Source: CAD feature listing. Evaluate the final solid. Frame: model axes, mm. A direction names the side the tool comes from. Give positions to 0.01 mm unless a question says otherwise; leave off trailing zeros. Order: outer loops, then holes, each group sorted by start corner. A loop starts at its lowest first (then second) coordinate and runs counter-clockwise, first axis right, second up.
from build123d import *

# Parameters (mm, degrees)
F0_W     = 25
F0_H     = 20
F0_R     = 4
F1_DEPTH = 10
F2_R     = 7.5
F3_DEPTH = 5
F4_W     = 14.7
F4_H     = 9.7
F4_R     = 4
F5_DEPTH = 0.5


with BuildPart() as f1:
    # F0 (on Top) → F1 (new body)
    with BuildSketch(Plane.XY):
        Rectangle(F0_W, F0_H)
        Circle(F0_R, mode=Mode.SUBTRACT)
    extrude(amount=F1_DEPTH)

    # F2 (on face) → F3 (cut)
    with BuildSketch(Plane.XY.offset(10)):
        Circle(F2_R)
    extrude(amount=-F3_DEPTH, mode=Mode.SUBTRACT)

    # F4 (on face) → F5 (join)
    with BuildSketch(Plane(origin=(0, 0, 0), x_dir=(1, 0, 0), z_dir=(0, 0, -1))):
        Rectangle(F4_W, F4_H)
        Circle(F4_R, mode=Mode.SUBTRACT)
    extrude(amount=F5_DEPTH)


solid = f1.part
(1) Section B-B, the plane y = 0. Return loops of the section in (x, z), plus the area to 3 significant figures.
(2) Section D-D, the plane x = -6. Return loops of the section in (y, z).
(3) Access query for faces 4 (the flat face through (0, -10, 5)), 5 (the flat face through (3, -3, 5)). Directions: +Z, -Z, +X, -X, +Y, -Y. A direction counts if a zero-diameter tool reaches every point of the face in a straight line with its end or side. Return the directions, or none.
(4) Section A-A, the plane x = 0. Return loops of the section in (y, z).
(5) Line query: line 1 along Y through (x, z) = (0, 3.7); line 2 along Y through (x, z) = (1.5, 7.5); line 3 along X through (y, z) = (0, 3.3). Output: solid intervals per line, ascending.
(6) Draft query along Y for faces 1 (the flat face through (0, 10, 5)), 2 (the flat face through (12.5, 0, 5)), 3 (the cylindrical face through (-0.867, 3.905, 2.288)). Return one class per face: +Y half, -Y half, draft (parallel to the pull), parting line (faces both ways), or undercut.
(7) Pin query (flat end, axial travel): pin 1 Ø12 at (x, y) = (0, 0) entering from +Z. Return the tip coordinate at first contact, or that it passes through.
(8) Section C-C, the plane z = 7.25. Return loops of the section in (x, y).
Checks:
1. outline: (-12.5, 0) - (-7.35, 0) - (-7.35, -0.5) - (-4, -0.5) - (-4, 5) - (-7.5, 5) - (-7.5, 10) - (-12.5, 10) - close; (4, -0.5) - (7.35, -0.5) - (7.35, 0) - (12.5, 0) - (12.5, 10) - (7.5, 10) - (7.5, 5) - (4, 5) - close
1. area: 138 mm2
2. outline: (-10, 0) - (-4.85, 0) - (-4.85, -0.5) - (4.85, -0.5) - (4.85, 0) - (10, 0) - (10, 10) - (4.5, 10) - (4.5, 5) - (-4.5, 5) - (-4.5, 10) - (-10, 10) - close
3. face 4: +Z, -Z, +X, -X, -Y
3. face 5: +Z
4. outline: (-10, 0) - (-4.85, 0) - (-4.85, -0.5) - (-4, -0.5) - (-4, 5) - (-7.5, 5) - (-7.5, 10) - (-10, 10) - close; (4, -0.5) - (4.85, -0.5) - (4.85, 0) - (10, 0) - (10, 10) - (7.5, 10) - (7.5, 5) - (4, 5) - close
5. line 1: y = -10 to -4, 4 to 10
5. line 2: y = -10 to -7.35, 7.35 to 10
5. line 3: x = -12.5 to -4, 4 to 12.5
6. face 1: +Y half
6. face 2: draft
6. face 3: undercut
7. pin 1: stops at z = 5
8. outline: (-12.5, -10) - (12.5, -10) - (12.5, 10) - (-12.5, 10) - close; hole circle Ø15 at (0, 0)
